Can you work these out from the model? Positions are in its coordinate system, mm. Give positions to 0.01 mm unless a question says otherwise; leave off trailing zeros. Answer as a JSON object with one key per item and string values.
```python
from build123d import *

# Parameters (mm, degrees)
SKETCH1_W           = 350
SKETCH1_H           = 350
BOSS_EXTRUDE1_DEPTH = 3
SKETCH2_R           = 3.75
SKETCH2_R_2         = 3.25
CUT_EXTRUDE1_DEPTH  = 3
SKETCH3_R           = 3.05
CUT_EXTRUDE2_DEPTH  = 3
SKETCH4_R           = 3
CUT_EXTRUDE3_DEPTH  = 3
SKETCH5_R           = 3.05
CUT_EXTRUDE4_DEPTH  = 3
CHAMFER1_SIZE       = 0.2


with BuildPart() as part:
    # Sketch1 → Boss-Extrude1 (new body)
    with BuildSketch(Plane(origin=(0, 0, 0), x_dir=(1, 0, 0), z_dir=(0, 1, 0))):
        Rectangle(SKETCH1_W, SKETCH1_H)
    extrude(amount=BOSS_EXTRUDE1_DEPTH)

    # Sketch2 → Cut-Extrude1 (cut)
    with BuildSketch(Plane(origin=(0, 3, 0), x_dir=(1, 0, 0), z_dir=(0, 1, 0))):
        with Locations(Location((0, -123.375, 0), (0, 0, 270))):
            Circle(SKETCH2_R)
        with Locations(Location((-150, -145, 0), (0, 0, 270))):
            Circle(SKETCH2_R_2)
        with Locations(Location((-150, 55, 0), (0, 0, 270))):
            Circle(SKETCH2_R_2)
        with Locations(Location((150, 55, 0), (0, 0, 270))):
            Circle(SKETCH2_R_2)
        with Locations(Location((150, -145, 0), (0, 0, 270))):
            Circle(SKETCH2_R_2)
    extrude(amount=-CUT_EXTRUDE1_DEPTH, mode=Mode.SUBTRACT)

    # Sketch3 → Cut-Extrude2 (cut)
    with BuildSketch(Plane(origin=(0, 3, 0), x_dir=(1, 0, 0), z_dir=(0, 1, 0))):
        with Locations(Location((-83.95, -62.901554786, 0), (0, 0, 270))):
            Circle(SKETCH3_R)
        with Locations(Location((83.95, -62.901554786, 0), (0, 0, 270))):
            Circle(SKETCH3_R)
    extrude(amount=-CUT_EXTRUDE2_DEPTH, mode=Mode.SUBTRACT)

    # Sketch4 → Cut-Extrude3 (cut)
    with BuildSketch(Plane(origin=(0, 3, 0), x_dir=(1, 0, 0), z_dir=(0, 1, 0))):
        with Locations(Location((-110.733018977, 165.110788036, 0), (0, 0, 270))):
            Circle(SKETCH4_R)
        with Locations(Location((-110.75, 22.110789044, 0), (0, 0, 270))):
            Circle(SKETCH4_R)
        with Locations(Location((110.749998438, 22.084486271, 0), (0, 0, 270))):
            Circle(SKETCH4_R)
        with Locations(Location((110.766979461, 165.084485263, 0), (0, 0, 270))):
            Circle(SKETCH4_R)
    extrude(amount=-CUT_EXTRUDE3_DEPTH, mode=Mode.SUBTRACT)

    # Sketch5 → Cut-Extrude4 (cut)
    with BuildSketch(Plane(origin=(0, 3, 0), x_dir=(1, 0, 0), z_dir=(0, 1, 0))):
        with Locations(Location((163.707635241, 83.030683972, 0), (0, 0, 270))):
            Circle(SKETCH5_R)
        with Locations(Location((127.458388125, 145.580683972, 0), (0, 0, 270))):
            Circle(SKETCH5_R)
    extrude(amount=-CUT_EXTRUDE4_DEPTH, mode=Mode.SUBTRACT)

    # Chamfer1
    chamfer1_edges = [part.edges().sort_by_distance(p)[0] for p in [
        (-175, 3, 0),
        (0, 3, 175),
        (150, 3, 141.75),
        (150, 0, 141.75),
        (150, 3, -58.25),
        (150, 0, -58.25),
        (-150, 3, -58.25),
        (-150, 0, -58.25),
        (-150, 3, 141.75),
        (-150, 0, 141.75),
        (0, 3, 119.625),
        (0, 0, 119.625),
        (-83.95, 3, 59.851554786),
        (-83.95, 0, 59.851554786),
        (83.95, 3, 59.851554786),
        (83.95, 0, 59.851554786),
        (175, 3, 0),
        (0, 0, 175),
        (-175, 0, 0),
        (110.766979461, 3, -168.084485263),
        (0, 0, -175),
        (110.766979461, 0, -168.084485263),
        (110.749998438, 3, -25.084486271),
        (110.749998438, 0, -25.084486271),
        (-110.75, 3, -25.110789044),
        (-110.75, 0, -25.110789044),
        (175, 0, 0),
        (-110.733018977, 3, -168.110788036),
        (-110.733018977, 0, -168.110788036),
        (163.707635241, 3, -86.080683972),
        (163.707635241, 0, -86.080683972),
        (127.458388125, 3, -148.630683972),
        (127.458388125, 0, -148.630683972),
        (0, 3, -175),
    ]]
    chamfer(chamfer1_edges, length=CHAMFER1_SIZE)


solid = part.part
```
1) Will this pin go through, and if not, where does the flat tip stop? pin 1 Ø4.5 at (x, z) = (0, 123.375) entering from -Y.
Answer list:
{"pin 1": "through"}
2) If we mould it in two halves opening along X, with no side actions, what happens to faces 1 (the flat face through (-2, 3, -2)), 2 (the cylindrical face through (-1.436, 1.518, 126.839))? For each: +X half, -X half, draft (parallel to the pull), parting line (faces both ways), or undercut.
Answer list:
{"face 1": "draft", "face 2": "undercut"}
3) Please list where these lines run through material, in increasing order: line 1 along X through (y, z) = (1.45, -55); line 2 along Z through (x, y) = (150, 1.25); line 3 along X through (y, z) = (2.55, -19.5). Write a range as from..to.
Answer list:
{"line 1": "-175..-153.25, -146.75..146.75, 153.25..175", "line 2": "-175..-58.25, -51.75..141.75, 148.25..175", "line 3": "-175..-112.23, -109.27..109.23, 112.27..175"}
